from build123d import *

# Parameters (mm, degrees)
SKETCH1_R           = 2
SKETCH1_R_2         = 3
BOSS_EXTRUDE1_DEPTH = 4.7625


with BuildPart() as part:
    # Sketch1 → Boss-Extrude1 (new body)
    with BuildSketch(Plane.XY):
        with BuildLine():
            Line((-14.25, -9.25), (-14.25, 13.536101268))
            ThreePointArc((-14.25, 13.536101268), (-13.704321085, 15.807449693), (-12.186390533, 17.583027341))
            ThreePointArc((-12.186390533, 17.583027341), (90, 50.75), (192.186390533, 17.583027341))
            ThreePointArc((192.186390533, 17.583027341), (193.704321085, 15.807449693), (194.25, 13.536101268))
            Line((194.25, 13.536101268), (194.25, -9.25))
            ThreePointArc((194.25, -9.25), (192.785533906, -12.785533906), (189.25, -14.25))
            Line((189.25, -14.25), (167.419194615, -14.25))
            ThreePointArc((167.419194615, -14.25), (165.851279553, -13.997803951), (164.441533284, -13.266656943))
            ThreePointArc((164.441533284, -13.266656943), (90, 11.316919489), (15.558466716, -13.266656943))
            ThreePointArc((15.558466716, -13.266656943), (14.148720447, -13.997803951), (12.580805385, -14.25))
            Line((12.580805385, -14.25), (-9.25, -14.25))
            ThreePointArc((-9.25, -14.25), (-12.785533906, -12.785533906), (-14.25, -9.25))
        make_face()
        with Locations((86, 44.6)):
            Circle(SKETCH1_R, mode=Mode.SUBTRACT)
        with Locations((86, 15.6)):
            Circle(SKETCH1_R, mode=Mode.SUBTRACT)
        with Locations((102, 44.6)):
            Circle(SKETCH1_R, mode=Mode.SUBTRACT)
        with Locations((102, 15.6)):
            Circle(SKETCH1_R, mode=Mode.SUBTRACT)
        with Locations((180, 0)):
            Circle(SKETCH1_R_2, mode=Mode.SUBTRACT)
        Circle(SKETCH1_R_2, mode=Mode.SUBTRACT)
        with Locations((4, 18.5)):
            Circle(SKETCH1_R_2, mode=Mode.SUBTRACT)
        with Locations((176, 18.5)):
            Circle(SKETCH1_R_2, mode=Mode.SUBTRACT)
    extrude(amount=BOSS_EXTRUDE1_DEPTH)


solid = part.part
Work out the finished part from the listing and answer in its coordinate system (mm). Give positions to 0.01 mm unless a question says otherwise; leave off trailing zeros. Write each loop counter-clockwise with the first axis right and the second up, starting at its lowest first coordinate (ties: lowest second). Pieces come first, ordered by that corner, then holes.
Q1. Straight lines are drawn through the part: L1, parallel to X at y = 1, z = 3.6; L2, parallel to X at y = 14, z = 0.55; L3, parallel to Y at x = 102, z = 1. For each, find the intervals that lie inside material, in ascending order.
Answer:
L1: x = -14.25 to -2.83, 2.83 to 40.27, 139.73 to 177.17, 182.83 to 194.25
L2: x = -14.23 to 84.8, 87.2 to 100.8, 103.2 to 194.23
L3: y = 10.74 to 13.6, 17.6 to 42.6, 46.6 to 50.34
Q2. The part is cut by section B-B on x = 86. Give the vertices of the cut face in (y, z).
Answer:
outline: (11.25, 0) - (13.6, 0) - (13.6, 4.76) - (11.25, 4.76) - close; (17.6, 0) - (42.6, 0) - (42.6, 4.76) - (17.6, 4.76) - close; (46.6, 0) - (50.7, 0) - (50.7, 4.76) - (46.6, 4.76) - close
Q3. The part is cut by section D-D on x = 132. Give the vertices of the cut face in (y, z), and give its area (3 significant figures).
Answer:
outline: (4.05, 0) - (45.6, 0) - (45.6, 4.76) - (4.05, 4.76) - close
area: 198 mm2
Q4. The part is cut by section C-C on x = 57.5. Give the vertices of the cut face in (y, z), and give its area (3 significant figures).
Answer:
outline: (7.02, 0) - (47.69, 0) - (47.69, 4.76) - (7.02, 4.76) - close
area: 194 mm2
Q5. For a pull along Y with two mould halves and no side action, classify faces 1 (the face through (193.689, 15.837, 2.348)), 2 (the face through (2, -14.25, 2)), 3 (the face through (3.35, 15.57, 2.35)) as released by +Y, released by -Y, zero draft, split by the parting line, or undercut.
Answer:
face 1: released by +Y
face 2: released by -Y
face 3: undercut
Q6. The part is cut by section A-A on z = 0.75. State how many separate pieces and enclosed holes the cut face has, and give its area (3 significant figures).
Answer:
separate pieces: 1
enclosed holes: 8
area: 8,430 mm2
Q7. Given pin 1 (1 mm diameter, centred on x = 35.5, z = 2.5, fed in from +Y), flat-ended and moving along its own axis, determine where the tip first touches the part or whether it passes through.
Answer:
pin 1: stops at y = 42.16
